Could you check a few things on this model? Use its own coordinates, in mm. A direction names the side the tool comes from. Round coordinates to 2 decimals unless told otherwise and drop trailing zeros. Loops run counter-clockwise (first coordinate to the right, second up) from the corner with the lowest first, then second, coordinate; pieces in that order, holes last. Notation, with made-up numbers: (77.25, -39) -> (106.25, -39) arc R20 ccw to (106.25, -1) -> close; hole circle Ø1 at (-2, 79). An arc over 180 degrees is marked (long way). Write each question's results on one line, items separated by ' | '. Start each with the question number.
1) We'd pull the mould along Y, two halves only. Please class faces 4 (the flat face through (44.763, 25.814, 12.522)), 5 (the flat face through (54, 0, 25.4)), 6 (the flat face through (18, -4.972, 26)): pulls with the +Y half, pulls with the -Y half, needs draft (parallel to the pull), parting line crosses it, or undercut.
2) Which directions (+Z, -Z, +X, -X, +Y, -Y) give clear straight access to the entire face, cutting with the end or side of a thin tool? Please do faces 1 (the cylindrical face through (-35.057, 1.543, 29.308)), 2 (the flat face through (18, 5.959, 26)), 3 (the flat face through (43.606, -26.126, 12.522)).
3) For P1, Ø1, axis at x = 67, z = 19, coming from the +Y side; P2, Ø3, axis at x = 17, z = 30.5, coming from the +Y side; P3, Ø5, axis at x = -2, z = 6.5, coming from the -Y side, each with a flat end and sliding along its axis, tell me the tip position at first contact or that it passes through.
4) If I drill on probe 1 along X at (y, z) = (0, 36.5); probe 2 along Y at (x, z) = (0, 37); probe 3 along X at (y, z) = (1.5, 17), over which ranges is the centre line in solid material (lowest first)?
5) Imagine slicing it at B-B, the plane z = 35. List the corners of the cut face in (x, y) for me.
6) Imagine slicing it at C-C, the plane y = -3.5. Give the number of separate pieces and of enclosed holes in the cut face, plus the area to 3 significant figures.
7) Imagine slicing it at A-A, the plane z = 6. List the corners of the cut face in (x, y) for me, plus the area to 3 significant figures.
from build123d import *

# Parameters (mm, degrees)
F1_DEPTH = 53.594
F2_DEPTH = 25.4
F3_R     = 5.08


with BuildPart() as f1:
    # F0 (on Top) → F1 (new body)
    with BuildSketch(Plane.XY):
        with BuildLine():
            Line((14.2938200345, 6.8228022219), (14.5426443405, 31.9357120423))
            ThreePointArc((14.5426443405, 31.9357120423), (-35.0892765953, 0.3476723709), (13.9069990558, -32.217597448))
            Line((13.9069990558, -32.217597448), (14.1558233618, -7.1046876277))
            ThreePointArc((14.1558233618, -7.1046876277), (-15.8379069236, 0.1569255107), (14.2938200345, 6.8228022219))
        make_face()
        with BuildLine():
            ThreePointArc((13.9069990558, -32.217597448), (29.3205448233, -19.2791042148), (35.0909989607, 0))
            ThreePointArc((35.0909989607, 0), (29.5101179725, 18.98765771), (14.5426443405, 31.9357120423))
            Line((14.5426443405, 31.9357120423), (14.2938200345, 6.8228022219))
            ThreePointArc((14.2938200345, 6.8228022219), (14.4908058573, 6.3937834608), (14.6749184523, 5.9590846408))
            Line((14.6749184523, 5.9590846408), (21.2465617806, 5.9590846408))
            Line((21.2465617806, 5.9590846408), (21.2465617806, 0))
            Line((21.2465617806, 0), (21.2465617806, -4.9716657959))
            Line((21.2465617806, -4.9716657959), (15.0381667949, -4.9716657959))
            ThreePointArc((15.0381667949, -4.9716657959), (14.6359048525, -6.0542720856), (14.1558233618, -7.1046876277))
            Line((14.1558233618, -7.1046876277), (13.9069990558, -32.217597448))
        make_face()
    extrude(amount=F1_DEPTH)

    # F0 (on Top) → F2 (join)
    with BuildSketch(Plane.XY):
        with BuildLine():
            ThreePointArc((14.5426443405, 31.9357120423), (29.5101179725, 18.98765771), (35.0909989607, 0))
            ThreePointArc((35.0909989607, 0), (29.3205448233, -19.2791042148), (13.9069990558, -32.217597448))
            Line((13.9069990558, -32.217597448), (74.1487775429, -19.8608903789))
            ThreePointArc((74.1487775429, -19.8608903789), (55.5140801332, 0), (74.1487775429, 19.8608903789))
            Line((74.1487775429, 19.8608903789), (14.5426443405, 31.9357120423))
        make_face()
        with BuildLine():
            ThreePointArc((95.3165463545, 0), (89.0324615704, 14.5131785208), (74.1487775429, 19.8608903789))
            Line((74.1487775429, 19.8608903789), (74.1487775429, 12.9542538791))
            ThreePointArc((74.1487775429, 12.9542538791), (84.1597843769, 9.6411114946), (88.4313343812, 0))
            ThreePointArc((88.4313343812, 0), (84.1597843769, -9.6411114946), (74.1487775429, -12.9542538791))
            Line((74.1487775429, -12.9542538791), (74.1487775429, -19.8608903789))
            ThreePointArc((74.1487775429, -19.8608903789), (89.0324615704, -14.5131785208), (95.3165463545, 0))
        make_face()
        with BuildLine():
            Line((74.1487775429, 12.9542538791), (74.1487775429, 19.8608903789))
            ThreePointArc((74.1487775429, 19.8608903789), (55.5140801332, 0), (74.1487775429, -19.8608903789))
            Line((74.1487775429, -19.8608903789), (74.1487775429, -12.9542538791))
            ThreePointArc((74.1487775429, -12.9542538791), (62.3992921066, 0), (74.1487775429, 12.9542538791))
        make_face()
    extrude(amount=F2_DEPTH)

    # F3
    f3_edges = [f1.edges().sort_by_distance(p)[0] for p in [
        (-13.906999, 32.217597, 53.594),
    ]]
    fillet(f3_edges, radius=F3_R)


solid = f1.part
Checked values:
1) face 4: pulls with the +Y half | face 5: needs draft | face 6: undercut
2) face 1: +Z | face 2: +Z, -Z | face 3: +Z, -Z, +X, -Y
3) P1: y = 21.41 | P2: y = 31.48 | P3: y = -35.09
4) probe 1: -35.09 to -15.84, 21.25 to 35.09 | probe 2: -35.09 to -15.84, 15.84 to 35.09 | probe 3: -35.06 to -15.77, 21.25 to 62.49, 88.34 to 95.26
5) outline: circle Ø70.18 at (0, 0); hole (14.67, 5.96) arc R15.84 ccw (long way) to (15.04, -4.97) -> (21.25, -4.97) -> (21.25, 5.96) -> close
6) separate pieces: 3 | enclosed holes: 0 | area: 2,650 mm^2
7) outline: (13.91, -32.22) -> (74.15, -19.86) arc R19.9 ccw (long way) to (74.15, 19.86) -> (14.54, 31.94) arc R35.09 ccw (long way) to start; hole (14.67, 5.96) arc R15.84 ccw (long way) to (15.04, -4.97) -> (21.25, -4.97) -> (21.25, 5.96) -> close; hole circle Ø26.03 at (75.42, 0) | area: 5,310 mm^2
